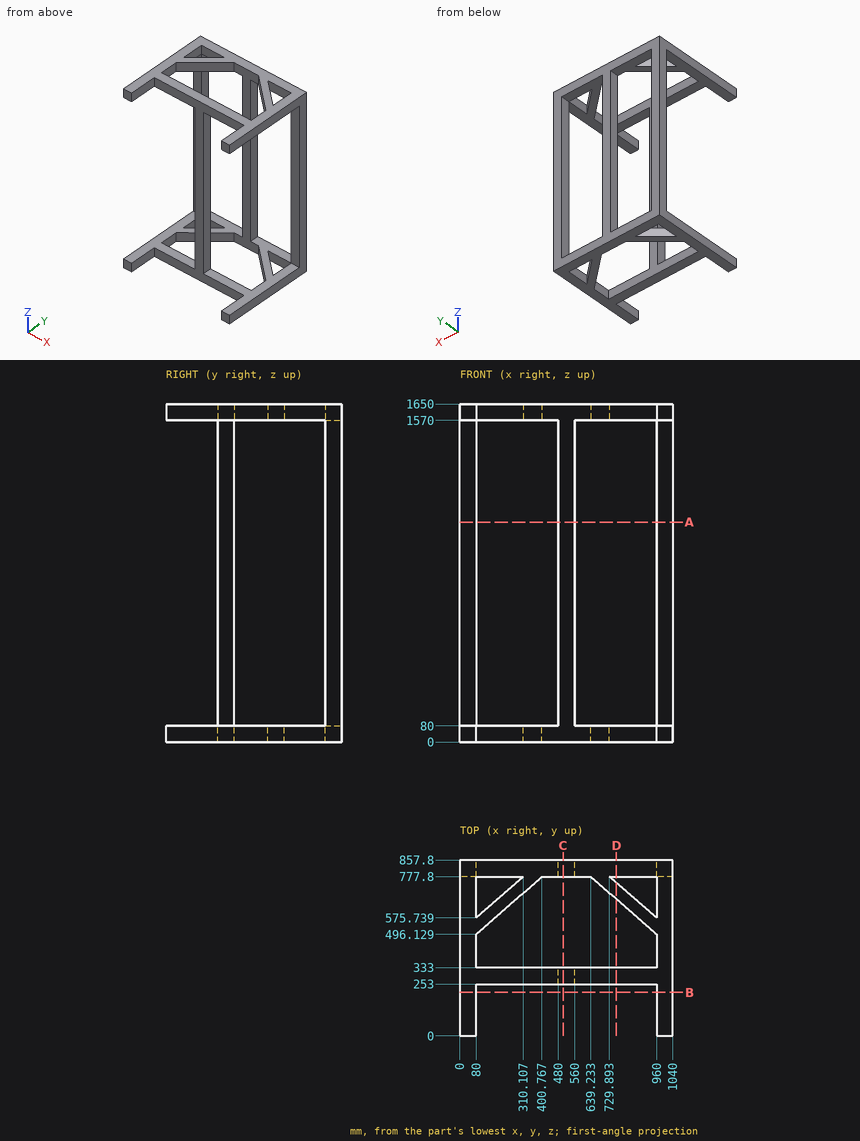
Job drawing, mm, ordinate dimensions from the low corner. One solid piece. Give positions to 0.01 mm unless a question says otherwise; leave off trailing zeros. Order: outer loops, then holes, each group sorted by start corner. A loop starts at its lowest first (then second) coordinate and runs counter-clockwise, first axis right, second up. Notation, with made-up numbers: M -4,71 L 12,71 A6 cw 12,78 Z; hole C -29.5,38.25 d7. An arc over 180 degrees is marked long. Put each result on its own line as item: value. Start each with the question number.
(1) Band-saw the part on A-A on z = 1074. Give the cut face in (x, y), then the cut area to 3 significant figures.
(2) Pin check, flat tips, straight feed: pin 1 Ø24 at (x, z) = (54, 807.5) entering from -Y; pin 2 Ø12 at (x, z) = (470, 1426.5) entering from +Y; pin 3 Ø24 at (y, z) = (294.5, 1104.5) entering from +X; pin 4 Ø10 at (x, z) = (527, 431.5) entering from -Y. Stop position of each tip, or through.
(3) Drill centre lines: L1, parallel to X at y = 794.5, z = 1434; L2, parallel to Z at x = 73.5, y = 602; L3, parallel to Y at x = 482.5, z = 933. Where is each one in solid material? Low to high. Write a range as [from, to].
(4) Band-saw the part on D-D on x = 764. Give the cut face in (y, z), then the cut area to 3 significant figures.
(5) Band-saw the part on C-C on x = 503.5. Give the cut face in (y, z).
(6) Band-saw the part on B-B on y = 212.5. Give the cut face in (x, z).
Results below:
1. outline: M 0,777.8 L 80,777.8 L 80,857.8 L 0,857.8 Z; M 480,253 L 560,253 L 560,333 L 480,333 Z; M 480,777.8 L 560,777.8 L 560,857.8 L 480,857.8 Z; M 960,777.8 L 1040,777.8 L 1040,857.8 L 960,857.8 Z
1. area: 25,600 mm2
2. pin 1: stops at y = 777.8
2. pin 2: passes through
2. pin 3: stops at x = 560
2. pin 4: stops at y = 253
3. L1: x = [0, 80], [480, 560], [960, 1040]
3. L2: z = [0, 80], [1570, 1650]
3. L3: y = [253, 333], [777.8, 857.8]
4. outline: M 253,0 L 333,0 L 333,80 L 253,80 Z; M 253,1570 L 333,1570 L 333,1650 L 253,1650 Z; M 668.24,0 L 747.85,0 L 747.85,80 L 668.24,80 Z; M 668.24,1570 L 747.85,1570 L 747.85,1650 L 668.24,1650 Z; M 777.8,0 L 857.8,0 L 857.8,80 L 777.8,80 Z; M 777.8,1570 L 857.8,1570 L 857.8,1650 L 777.8,1650 Z
4. area: 38,300 mm2
5. outline: M 253,0 L 333,0 L 333,1650 L 253,1650 Z; M 777.8,0 L 857.8,0 L 857.8,1650 L 777.8,1650 Z
6. outline: M 0,0 L 80,0 L 80,80 L 0,80 Z; M 0,1570 L 80,1570 L 80,1650 L 0,1650 Z; M 960,0 L 1040,0 L 1040,80 L 960,80 Z; M 960,1570 L 1040,1570 L 1040,1650 L 960,1650 Z
